Here's how the part is built. I have some questions about the finished solid (model axes, mm). Coordinates: 2 decimals unless noted, no trailing zeros. Order: outer loops, then holes, each group sorted by start corner. A loop starts at its lowest first (then second) coordinate and runs counter-clockwise, first axis right, second up. Notation, with made-up numbers: (80, 13) - (101, 13) arc R29 cw to (101, 50) - close; hole circle Ø7 at (21.5, -30). An arc over 180 degrees is marked (long way). Answer in a Markdown table with one row per item. Add a question column.
Item 1: Thinking about a two-plate mould opening in Y: for faces 1 (the cylindrical face through (62.903, 35.891, 1.017)), 2 (the flat face through (-118, 100, 0)), which applies, +Y half, -Y half, draft (parallel to the pull), parting line (faces both ways), or undercut?
Item 2: I want a section at B-B (z = 1.5). Count the separate pieces of the cut face and the enclosed holes in it, plus the area to 3 significant figures.
Item 3: I want a section at A-A (x = 74.5). Please give me the cut outline in (y, z), plus the area to 3 significant figures.
Item 4: If I drill on line 1 along Y through (x, z) = (-300, 0.6); line 2 along X through (y, z) = (31.5, 1.8); line 3 along X through (y, z) = (31, 1.3), over which ranges is the centre line in solid material (lowest first)? Write a range as from..to.
Item 5: I want a section at C-C (x = -297.5). Please give me the cut outline in (y, z), plus the area to 3 significant figures.
Autodesk Inventor part; units mm, degrees
ref_plane "YZ Plane" through (0, 0, 0) normal (1, 0, 0) x (0, 1, 0)
ref_plane "XZ Plane" through (0, 0, 0) normal (0, 1, 0) x (-1, 0, 0)
ref_plane "XY Plane" through (0, 0, 0) normal (0, 0, 1) x (1, 0, 0)
sketch "Sketch1" plane through (0, 0, 0) normal (0, 0, 1) x (1, 0, 0)
  line L0 (-363.5144, 243.2472) -> (135.0368, 243.2472)
  line L1 (135.0368, 243.2472) -> (135.0368, -47.8114)
  line L2 (135.0368, -47.8114) -> (-363.5144, -47.8114)
  line L3 (-363.5144, -47.8114) -> (-363.5144, 243.2472)
  point P0 (0, 0)
  dimension "d0" = 498.5512
  dimension "d1" = 291.0586
extrude "Extrusion1" add sketch "Sketch1" along normal blind 2.0066
sketch "Sketch2" plane through (0, 0, 2.0066) normal (0, 0, 1) x (1, 0, 0)
  circle A0 centre (82.6198, 35.0228) radius 19.7358
  circle A1 centre (66.3698, 18.7728) radius 1.25
  line L0 (385.8263, -153.0596) -> (385.8263, 254.4224)
  line L1 (-77.3983, -47.0364) -> (620.5734, -47.0364)
  circle A2 centre (66.3698, 51.2728) radius 1.25
  circle A3 centre (98.8698, 18.7728) radius 1.25
  circle A4 centre (98.8698, 51.2728) radius 1.25
  point P0 (385.8263, -47.0364)
  dimension "d4" = 39.4716
  dimension "d5" = 2.5
  dimension "d11" = 32.5
  dimension "d14" = 32.5
  dimension "d17" = 16.25
  dimension "d18" = 16.25
extrude "Joystick 1" cut sketch "Sketch2" against normal blind 2.0066
sketch "Sketch3" plane through (1.6331, 0.1353, 2.0066) normal (0, 0, 1) x (1, 0, 0)
  circle A0 centre (-301.0067, 37.2418) radius 19.7358
  circle A1 centre (-317.2567, 20.9918) radius 1.25
  line L0 (0, -106.0232) -> (0, 301.4589)
  line L1 (-463.2246, 0) -> (234.7471, 0)
  circle A2 centre (-317.2567, 53.4918) radius 1.25
  circle A3 centre (-284.7567, 20.9918) radius 1.25
  circle A4 centre (-284.7567, 53.4918) radius 1.25
  point P0 (0, 0)
  dimension "d30" = 39.4716
  dimension "d28" = 2.5
  dimension "d22" = 32.5
  dimension "d21" = 32.5
  dimension "d27" = 16.25
  dimension "d29" = 16.25
extrude "Joystick 2" cut sketch "Sketch3" against normal blind 2.0066
sketch "Sketch4" plane through (0, 0, 2.0066) normal (0, 0, 1) x (1, 0, 0)
  circle A0 centre (-117.2987, 153.872) radius 21.5
  circle A1 centre (-117.2987, 179.272) radius 1.75
  circle A2 centre (-139.2957, 141.172) radius 1.75
  circle A3 centre (-95.3016, 141.172) radius 1.75
  point P0 (0, 0)
  dimension "d34" = 43
  dimension "d35" = 25.4
  dimension "d36" = 3.5
  dimension "d39" = 360
extrude "Throttle Encoder" cut sketch "Sketch4" against normal blind 2.0066
properties part number "Panel"
Values follow:
| question | item | result |
|---|---|---|
| 1 | face 1 | undercut |
| 1 | face 2 | draft |
| 2 | separate pieces | 1 |
| 2 | enclosed holes | 14 |
| 2 | area | 141,000 mm^2 |
| 3 | outline | (-47.81, 0) - (17.03, 0) - (17.03, 2.01) - (-47.81, 2.01) - close; (53.01, 0) - (243.25, 0) - (243.25, 2.01) - (53.01, 2.01) - close |
| 3 | area | 512 mm^2 |
| 4 | line 1 | y = -47.81..17.65, 57.1..243.25 |
| 4 | line 2 | x = -363.51..-318.21, -280.53..63.2, 102.04..135.04 |
| 4 | line 3 | x = -363.51..-318.05, -280.7..63.3, 101.94..135.04 |
| 5 | outline | (-47.81, 0) - (17.73, 0) - (17.73, 2.01) - (-47.81, 2.01) - close; (57.02, 0) - (243.25, 0) - (243.25, 2.01) - (57.02, 2.01) - close |
| 5 | area | 505 mm^2 |
